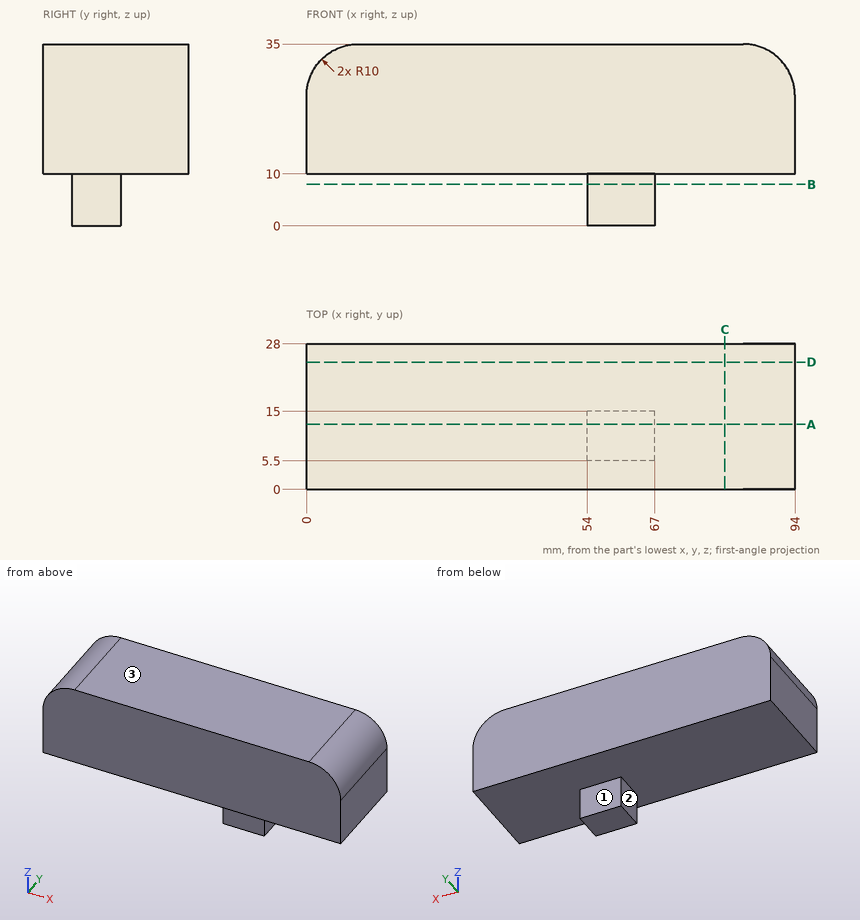
Study the drawing (mm; zero at the part's minimum x, y, z) and answer. A direction names the side the tool comes from. Coordinates: 2 decimals unless noted, no trailing zeros. Write each loop counter-clockwise with the first axis right and the second up, starting at its lowest first coordinate (ties: lowest second). Pieces come first, ordered by that corner, then holes. Notation, with made-up numbers: M 68.25,28.5 L 97.25,28.5 A22 ccw 97.25,62.5 Z; hole C -26,-27 d3. An arc over 180 degrees is marked long. Use a Markdown table: item, result. Add a question column.
1. Which of the six approach directions +Z, -Z, +X, -X, +Y, -Y give full straight-line access (tool end or side, diameter ignored) to the marked faces 1, 2 and 3?
2. Given P1, Ø1, axis at y = 22, z = 28.5, coming from the +X side; P2, Ø8, axis at x = 63, z = 6.5, coming from the -Y side; P3, Ø5, axis at y = 11, z = 4, coming from the -X side; P4, Ø2, axis at y = 10, z = 29, coming from the -X side, each flat-ended and moving along its own axis, determine where each tip first touches the part or whether it passes through.
3. Section D-D (y = 24.5) is taken. Give the vertices of the cut face in (x, z), plus the area to 3 significant figures.
4. Straight lines are drawn through the part: line 1 along X through (y, z) = (7.5, 5); line 2 along Z through (x, y) = (14, 10.5); line 3 along X through (y, z) = (26, 25.5). For each, find the intervals that lie inside material, in ascending order. Write a range as [from, to].
5. Section A-A (y = 12.5) is taken. Give the vertices of the cut face in (x, z).
6. Section C-C (x = 80.5) is taken. Give the vertices of the cut face in (y, z).
7. Section B-B (z = 8) is taken. Give the vertices of the cut face in (x, y).
Data:
| question | item | result |
|---|---|---|
| 1 | face 1 | -Z, +X, -X, +Y |
| 1 | face 2 | -Z, -X, +Y, -Y |
| 1 | face 3 | +Z, +X, -X, +Y, -Y |
| 2 | P1 | stops at x = 93.54 |
| 2 | P2 | stops at y = 0 |
| 2 | P3 | stops at x = 54 |
| 2 | P4 | stops at x = 0.46 |
| 3 | outline | M 0,10 L 94,10 L 94,25 A10 ccw 84,35 L 10,35 A10 ccw 0,25 Z |
| 3 | area | 2,310 mm2 |
| 4 | line 1 | x = [54, 67] |
| 4 | line 2 | z = [10, 35] |
| 4 | line 3 | x = [0.01, 93.99] |
| 5 | outline | M 0,10 L 54,10 L 54,0 L 67,0 L 67,10 L 94,10 L 94,25 A10 ccw 84,35 L 10,35 A10 ccw 0,25 Z |
| 6 | outline | M 0,10 L 28,10 L 28,35 L 0,35 Z |
| 7 | outline | M 54,5.5 L 67,5.5 L 67,15 L 54,15 Z |
